Verification items for the finished model (mm, model axes). Round coordinates to 2 decimals unless told otherwise and drop trailing zeros. One line per item, written item: value.
from build123d import *

# Parameters (mm, degrees)
SKETCH_1_W          = 9
SKETCH_1_H          = 6.5
EXTRUDE_1_DEPTH     = 590
SKETCH_2_W          = 2
SKETCH_2_H          = 1
CUT_EXTRUDE_1_DEPTH = 610
CUT_EXTRUDE_2_REACH = 592.104
SKETCH_3_R          = 1.5
SKETCH_4_R          = 1.656535544
CUT_EXTRUDE_3_DEPTH = 10


with BuildPart() as part:
    # 草图1 → 凸台-拉伸1 (new body)
    with BuildSketch(Plane.XY):
        with Locations((-4.5, 3.25)):
            Rectangle(SKETCH_1_W, SKETCH_1_H)
    extrude(amount=EXTRUDE_1_DEPTH)

    # 草图2 → 切除-拉伸1 (cut)
    with BuildSketch(Plane(origin=(0, 0, 0), x_dir=(-1, 0, 0), z_dir=(0, 0, -1))):
        with Locations((1, 5)):
            Rectangle(SKETCH_2_W, SKETCH_2_H)
        with Locations((8, 5)):
            Rectangle(SKETCH_2_W, SKETCH_2_H)
    extrude(amount=-CUT_EXTRUDE_1_DEPTH, mode=Mode.SUBTRACT)

    # 草图3 → 切除-拉伸2 (cut, up to next)
    with BuildSketch(Plane(origin=(0, 6.5, 0), x_dir=(1, 0, 0), z_dir=(0, 1, 0)), mode=Mode.PRIVATE) as cut_extrude_2_sk1:
        with Locations(Location((-4.5, -5, 0), (0, 0, 180))):
            Circle(SKETCH_3_R)
    cut_extrude_2_tool1 = extrude(cut_extrude_2_sk1.sketch, amount=-CUT_EXTRUDE_2_REACH, mode=Mode.PRIVATE) & part.part
    # 草图3 → 切除-拉伸2 (cut, up to next)
    with BuildSketch(Plane(origin=(0, 6.5, 0), x_dir=(1, 0, 0), z_dir=(0, 1, 0)), mode=Mode.PRIVATE) as cut_extrude_2_sk2:
        with Locations(Location((-4.5, -25, 0), (0, 0, 180))):
            Circle(SKETCH_3_R)
    cut_extrude_2_tool2 = extrude(cut_extrude_2_sk2.sketch, amount=-CUT_EXTRUDE_2_REACH, mode=Mode.PRIVATE) & part.part
    # 草图3 → 切除-拉伸2 (cut, up to next)
    with BuildSketch(Plane(origin=(0, 6.5, 0), x_dir=(1, 0, 0), z_dir=(0, 1, 0)), mode=Mode.PRIVATE) as cut_extrude_2_sk3:
        with Locations(Location((-4.5, -45, 0), (0, 0, 180))):
            Circle(SKETCH_3_R)
    cut_extrude_2_tool3 = extrude(cut_extrude_2_sk3.sketch, amount=-CUT_EXTRUDE_2_REACH, mode=Mode.PRIVATE) & part.part
    # 草图3 → 切除-拉伸2 (cut, up to next)
    with BuildSketch(Plane(origin=(0, 6.5, 0), x_dir=(1, 0, 0), z_dir=(0, 1, 0)), mode=Mode.PRIVATE) as cut_extrude_2_sk4:
        with Locations(Location((-4.5, -65, 0), (0, 0, 180))):
            Circle(SKETCH_3_R)
    cut_extrude_2_tool4 = extrude(cut_extrude_2_sk4.sketch, amount=-CUT_EXTRUDE_2_REACH, mode=Mode.PRIVATE) & part.part
    # 草图3 → 切除-拉伸2 (cut, up to next)
    with BuildSketch(Plane(origin=(0, 6.5, 0), x_dir=(1, 0, 0), z_dir=(0, 1, 0)), mode=Mode.PRIVATE) as cut_extrude_2_sk5:
        with Locations(Location((-4.5, -85, 0), (0, 0, 180))):
            Circle(SKETCH_3_R)
    cut_extrude_2_tool5 = extrude(cut_extrude_2_sk5.sketch, amount=-CUT_EXTRUDE_2_REACH, mode=Mode.PRIVATE) & part.part
    # 草图3 → 切除-拉伸2 (cut, up to next)
    with BuildSketch(Plane(origin=(0, 6.5, 0), x_dir=(1, 0, 0), z_dir=(0, 1, 0)), mode=Mode.PRIVATE) as cut_extrude_2_sk6:
        with Locations(Location((-4.5, -105, 0), (0, 0, 180))):
            Circle(SKETCH_3_R)
    cut_extrude_2_tool6 = extrude(cut_extrude_2_sk6.sketch, amount=-CUT_EXTRUDE_2_REACH, mode=Mode.PRIVATE) & part.part
    # 草图3 → 切除-拉伸2 (cut, up to next)
    with BuildSketch(Plane(origin=(0, 6.5, 0), x_dir=(1, 0, 0), z_dir=(0, 1, 0)), mode=Mode.PRIVATE) as cut_extrude_2_sk7:
        with Locations(Location((-4.5, -125, 0), (0, 0, 180))):
            Circle(SKETCH_3_R)
    cut_extrude_2_tool7 = extrude(cut_extrude_2_sk7.sketch, amount=-CUT_EXTRUDE_2_REACH, mode=Mode.PRIVATE) & part.part
    # 草图3 → 切除-拉伸2 (cut, up to next)
    with BuildSketch(Plane(origin=(0, 6.5, 0), x_dir=(1, 0, 0), z_dir=(0, 1, 0)), mode=Mode.PRIVATE) as cut_extrude_2_sk8:
        with Locations(Location((-4.5, -145, 0), (0, 0, 180))):
            Circle(SKETCH_3_R)
    cut_extrude_2_tool8 = extrude(cut_extrude_2_sk8.sketch, amount=-CUT_EXTRUDE_2_REACH, mode=Mode.PRIVATE) & part.part
    # 草图3 → 切除-拉伸2 (cut, up to next)
    with BuildSketch(Plane(origin=(0, 6.5, 0), x_dir=(1, 0, 0), z_dir=(0, 1, 0)), mode=Mode.PRIVATE) as cut_extrude_2_sk9:
        with Locations(Location((-4.5, -165, 0), (0, 0, 180))):
            Circle(SKETCH_3_R)
    cut_extrude_2_tool9 = extrude(cut_extrude_2_sk9.sketch, amount=-CUT_EXTRUDE_2_REACH, mode=Mode.PRIVATE) & part.part
    # 草图3 → 切除-拉伸2 (cut, up to next)
    with BuildSketch(Plane(origin=(0, 6.5, 0), x_dir=(1, 0, 0), z_dir=(0, 1, 0)), mode=Mode.PRIVATE) as cut_extrude_2_sk10:
        with Locations(Location((-4.5, -185, 0), (0, 0, 180))):
            Circle(SKETCH_3_R)
    cut_extrude_2_tool10 = extrude(cut_extrude_2_sk10.sketch, amount=-CUT_EXTRUDE_2_REACH, mode=Mode.PRIVATE) & part.part
    # 草图3 → 切除-拉伸2 (cut, up to next)
    with BuildSketch(Plane(origin=(0, 6.5, 0), x_dir=(1, 0, 0), z_dir=(0, 1, 0)), mode=Mode.PRIVATE) as cut_extrude_2_sk11:
        with Locations(Location((-4.5, -205, 0), (0, 0, 180))):
            Circle(SKETCH_3_R)
    cut_extrude_2_tool11 = extrude(cut_extrude_2_sk11.sketch, amount=-CUT_EXTRUDE_2_REACH, mode=Mode.PRIVATE) & part.part
    # 草图3 → 切除-拉伸2 (cut, up to next)
    with BuildSketch(Plane(origin=(0, 6.5, 0), x_dir=(1, 0, 0), z_dir=(0, 1, 0)), mode=Mode.PRIVATE) as cut_extrude_2_sk12:
        with Locations(Location((-4.5, -225, 0), (0, 0, 180))):
            Circle(SKETCH_3_R)
    cut_extrude_2_tool12 = extrude(cut_extrude_2_sk12.sketch, amount=-CUT_EXTRUDE_2_REACH, mode=Mode.PRIVATE) & part.part
    # 草图3 → 切除-拉伸2 (cut, up to next)
    with BuildSketch(Plane(origin=(0, 6.5, 0), x_dir=(1, 0, 0), z_dir=(0, 1, 0)), mode=Mode.PRIVATE) as cut_extrude_2_sk13:
        with Locations(Location((-4.5, -245, 0), (0, 0, 180))):
            Circle(SKETCH_3_R)
    cut_extrude_2_tool13 = extrude(cut_extrude_2_sk13.sketch, amount=-CUT_EXTRUDE_2_REACH, mode=Mode.PRIVATE) & part.part
    # 草图3 → 切除-拉伸2 (cut, up to next)
    with BuildSketch(Plane(origin=(0, 6.5, 0), x_dir=(1, 0, 0), z_dir=(0, 1, 0)), mode=Mode.PRIVATE) as cut_extrude_2_sk14:
        with Locations(Location((-4.5, -265, 0), (0, 0, 180))):
            Circle(SKETCH_3_R)
    cut_extrude_2_tool14 = extrude(cut_extrude_2_sk14.sketch, amount=-CUT_EXTRUDE_2_REACH, mode=Mode.PRIVATE) & part.part
    # 草图3 → 切除-拉伸2 (cut, up to next)
    with BuildSketch(Plane(origin=(0, 6.5, 0), x_dir=(1, 0, 0), z_dir=(0, 1, 0)), mode=Mode.PRIVATE) as cut_extrude_2_sk15:
        with Locations(Location((-4.5, -285, 0), (0, 0, 180))):
            Circle(SKETCH_3_R)
    cut_extrude_2_tool15 = extrude(cut_extrude_2_sk15.sketch, amount=-CUT_EXTRUDE_2_REACH, mode=Mode.PRIVATE) & part.part
    # 草图3 → 切除-拉伸2 (cut, up to next)
    with BuildSketch(Plane(origin=(0, 6.5, 0), x_dir=(1, 0, 0), z_dir=(0, 1, 0)), mode=Mode.PRIVATE) as cut_extrude_2_sk16:
        with Locations(Location((-4.5, -305, 0), (0, 0, 180))):
            Circle(SKETCH_3_R)
    cut_extrude_2_tool16 = extrude(cut_extrude_2_sk16.sketch, amount=-CUT_EXTRUDE_2_REACH, mode=Mode.PRIVATE) & part.part
    # 草图3 → 切除-拉伸2 (cut, up to next)
    with BuildSketch(Plane(origin=(0, 6.5, 0), x_dir=(1, 0, 0), z_dir=(0, 1, 0)), mode=Mode.PRIVATE) as cut_extrude_2_sk17:
        with Locations(Location((-4.5, -325, 0), (0, 0, 180))):
            Circle(SKETCH_3_R)
    cut_extrude_2_tool17 = extrude(cut_extrude_2_sk17.sketch, amount=-CUT_EXTRUDE_2_REACH, mode=Mode.PRIVATE) & part.part
    # 草图3 → 切除-拉伸2 (cut, up to next)
    with BuildSketch(Plane(origin=(0, 6.5, 0), x_dir=(1, 0, 0), z_dir=(0, 1, 0)), mode=Mode.PRIVATE) as cut_extrude_2_sk18:
        with Locations(Location((-4.5, -345, 0), (0, 0, 180))):
            Circle(SKETCH_3_R)
    cut_extrude_2_tool18 = extrude(cut_extrude_2_sk18.sketch, amount=-CUT_EXTRUDE_2_REACH, mode=Mode.PRIVATE) & part.part
    # 草图3 → 切除-拉伸2 (cut, up to next)
    with BuildSketch(Plane(origin=(0, 6.5, 0), x_dir=(1, 0, 0), z_dir=(0, 1, 0)), mode=Mode.PRIVATE) as cut_extrude_2_sk19:
        with Locations(Location((-4.5, -365, 0), (0, 0, 180))):
            Circle(SKETCH_3_R)
    cut_extrude_2_tool19 = extrude(cut_extrude_2_sk19.sketch, amount=-CUT_EXTRUDE_2_REACH, mode=Mode.PRIVATE) & part.part
    # 草图3 → 切除-拉伸2 (cut, up to next)
    with BuildSketch(Plane(origin=(0, 6.5, 0), x_dir=(1, 0, 0), z_dir=(0, 1, 0)), mode=Mode.PRIVATE) as cut_extrude_2_sk20:
        with Locations(Location((-4.5, -385, 0), (0, 0, 180))):
            Circle(SKETCH_3_R)
    cut_extrude_2_tool20 = extrude(cut_extrude_2_sk20.sketch, amount=-CUT_EXTRUDE_2_REACH, mode=Mode.PRIVATE) & part.part
    # 草图3 → 切除-拉伸2 (cut, up to next)
    with BuildSketch(Plane(origin=(0, 6.5, 0), x_dir=(1, 0, 0), z_dir=(0, 1, 0)), mode=Mode.PRIVATE) as cut_extrude_2_sk21:
        with Locations(Location((-4.5, -405, 0), (0, 0, 180))):
            Circle(SKETCH_3_R)
    cut_extrude_2_tool21 = extrude(cut_extrude_2_sk21.sketch, amount=-CUT_EXTRUDE_2_REACH, mode=Mode.PRIVATE) & part.part
    # 草图3 → 切除-拉伸2 (cut, up to next)
    with BuildSketch(Plane(origin=(0, 6.5, 0), x_dir=(1, 0, 0), z_dir=(0, 1, 0)), mode=Mode.PRIVATE) as cut_extrude_2_sk22:
        with Locations(Location((-4.5, -425, 0), (0, 0, 180))):
            Circle(SKETCH_3_R)
    cut_extrude_2_tool22 = extrude(cut_extrude_2_sk22.sketch, amount=-CUT_EXTRUDE_2_REACH, mode=Mode.PRIVATE) & part.part
    # 草图3 → 切除-拉伸2 (cut, up to next)
    with BuildSketch(Plane(origin=(0, 6.5, 0), x_dir=(1, 0, 0), z_dir=(0, 1, 0)), mode=Mode.PRIVATE) as cut_extrude_2_sk23:
        with Locations(Location((-4.5, -445, 0), (0, 0, 180))):
            Circle(SKETCH_3_R)
    cut_extrude_2_tool23 = extrude(cut_extrude_2_sk23.sketch, amount=-CUT_EXTRUDE_2_REACH, mode=Mode.PRIVATE) & part.part
    add(cut_extrude_2_tool1.solids().sort_by_distance((-4.5, 6.5, 5))[0], mode=Mode.SUBTRACT)
    add(cut_extrude_2_tool2.solids().sort_by_distance((-4.5, 6.5, 25))[0], mode=Mode.SUBTRACT)
    add(cut_extrude_2_tool3.solids().sort_by_distance((-4.5, 6.5, 45))[0], mode=Mode.SUBTRACT)
    add(cut_extrude_2_tool4.solids().sort_by_distance((-4.5, 6.5, 65))[0], mode=Mode.SUBTRACT)
    add(cut_extrude_2_tool5.solids().sort_by_distance((-4.5, 6.5, 85))[0], mode=Mode.SUBTRACT)
    add(cut_extrude_2_tool6.solids().sort_by_distance((-4.5, 6.5, 105))[0], mode=Mode.SUBTRACT)
    add(cut_extrude_2_tool7.solids().sort_by_distance((-4.5, 6.5, 125))[0], mode=Mode.SUBTRACT)
    add(cut_extrude_2_tool8.solids().sort_by_distance((-4.5, 6.5, 145))[0], mode=Mode.SUBTRACT)
    add(cut_extrude_2_tool9.solids().sort_by_distance((-4.5, 6.5, 165))[0], mode=Mode.SUBTRACT)
    add(cut_extrude_2_tool10.solids().sort_by_distance((-4.5, 6.5, 185))[0], mode=Mode.SUBTRACT)
    add(cut_extrude_2_tool11.solids().sort_by_distance((-4.5, 6.5, 205))[0], mode=Mode.SUBTRACT)
    add(cut_extrude_2_tool12.solids().sort_by_distance((-4.5, 6.5, 225))[0], mode=Mode.SUBTRACT)
    add(cut_extrude_2_tool13.solids().sort_by_distance((-4.5, 6.5, 245))[0], mode=Mode.SUBTRACT)
    add(cut_extrude_2_tool14.solids().sort_by_distance((-4.5, 6.5, 265))[0], mode=Mode.SUBTRACT)
    add(cut_extrude_2_tool15.solids().sort_by_distance((-4.5, 6.5, 285))[0], mode=Mode.SUBTRACT)
    add(cut_extrude_2_tool16.solids().sort_by_distance((-4.5, 6.5, 305))[0], mode=Mode.SUBTRACT)
    add(cut_extrude_2_tool17.solids().sort_by_distance((-4.5, 6.5, 325))[0], mode=Mode.SUBTRACT)
    add(cut_extrude_2_tool18.solids().sort_by_distance((-4.5, 6.5, 345))[0], mode=Mode.SUBTRACT)
    add(cut_extrude_2_tool19.solids().sort_by_distance((-4.5, 6.5, 365))[0], mode=Mode.SUBTRACT)
    add(cut_extrude_2_tool20.solids().sort_by_distance((-4.5, 6.5, 385))[0], mode=Mode.SUBTRACT)
    add(cut_extrude_2_tool21.solids().sort_by_distance((-4.5, 6.5, 405))[0], mode=Mode.SUBTRACT)
    add(cut_extrude_2_tool22.solids().sort_by_distance((-4.5, 6.5, 425))[0], mode=Mode.SUBTRACT)
    add(cut_extrude_2_tool23.solids().sort_by_distance((-4.5, 6.5, 445))[0], mode=Mode.SUBTRACT)

    # 草图4 → 切除-拉伸3 (cut)
    with BuildSketch(Plane(origin=(0, 6.5, 0), x_dir=(1, 0, 0), z_dir=(0, 1, 0))):
        with Locations(Location((-4.5, -465, 0), (0, 0, 180))):
            Circle(SKETCH_4_R)
        with Locations(Location((-4.5, -485, 0), (0, 0, 180))):
            Circle(SKETCH_4_R)
        with Locations(Location((-4.5, -505, 0), (0, 0, 180))):
            Circle(SKETCH_4_R)
        with Locations(Location((-4.5, -525, 0), (0, 0, 180))):
            Circle(SKETCH_4_R)
        with Locations(Location((-4.5, -545, 0), (0, 0, 180))):
            Circle(SKETCH_4_R)
        with Locations(Location((-4.5, -565, 0), (0, 0, 180))):
            Circle(SKETCH_4_R)
        with Locations(Location((-4.5, -585, 0), (0, 0, 180))):
            Circle(SKETCH_4_R)
    extrude(amount=-CUT_EXTRUDE_3_DEPTH, mode=Mode.SUBTRACT)


solid = part.part
(1) Thickness scan on L1, parallel to X at y = 3.25, z = 345; L2, parallel to X at y = 3.75, z = 585; L3, parallel to Y at x = -7.5, z = 49.5. Record the ranges inside material, lowest first. Write a range as from..to.
Completed:
L1: x = -9..-6, -3..0
L2: x = -9..-6.16, -2.84..0
L3: y = 0..4.5, 5.5..6.5
(2) Sectioned sample at A-A on y = 1.5. Count the separate pieces of the cut face and the enclosed holes in it, and give its area (3 significant figures).
Completed:
separate pieces: 1
enclosed holes: 30
area: 5,090 mm^2
(3) Depth check by flat-ended pin: pin 1 Ø2 at (x, z) = (-4.5, 485) entering from +Y. Enter the tip coordinate at first touch or a pass-through.
Completed:
pin 1: passes through
